```python
from build123d import *

# Parameters (mm, degrees)
SKETCH_1_R          = 17.5
EXTRUDE_1_DEPTH     = 15
SKETCH_2_R          = 1.5
CUT_EXTRUDE_1_DEPTH = 5
SKETCH_4_R          = 3
CUT_EXTRUDE_2_DEPTH = 20
SKETCH_5_R          = 1.5
CUT_EXTRUDE_3_DEPTH = 6
CHAMFER_1_SIZE      = 1.5
SKETCH_6_R          = 6.5
SKETCH_6_R_2        = 3.996615851
CUT_EXTRUDE_4_DEPTH = 3
SKETCH_7_R          = 3.996615851
SKETCH_7_R_2        = 3
EXTRUDE_2_DEPTH     = 1


with BuildPart() as part:
    # 草图1 → 凸台-拉伸1 (new body)
    with BuildSketch(Plane.XY):
        Circle(SKETCH_1_R)
    extrude(amount=EXTRUDE_1_DEPTH)

    # 草图2 → 切除-拉伸1 (cut)
    with BuildSketch(Plane(origin=(0, 0, 0), x_dir=(-1, 0, 0), z_dir=(0, 0, -1))):
        with Locations((0, -8)):
            Circle(SKETCH_2_R)
        with Locations((-8, 0)):
            Circle(SKETCH_2_R)
        with Locations((0, 8)):
            Circle(SKETCH_2_R)
        with Locations((8, 0)):
            Circle(SKETCH_2_R)
    extrude(amount=-CUT_EXTRUDE_1_DEPTH, mode=Mode.SUBTRACT)

    # 草图3 → 切除-旋转1 (revolve, cut)
    with BuildSketch(Plane(origin=(0, 0, 0), x_dir=(1, 0, 0), z_dir=(0, 1, 0))):
        Polygon((13.284433797, -10), (13.284433797, -9.953144571), (13.284433797, -9.453144571), (17.969347124, -9.453144571), (17.969347124, -10), align=None)
    revolve(axis=Axis((0, 0, 0), (0, 0, 1)), mode=Mode.SUBTRACT)

    # 草图4 → 切除-拉伸2 (cut)
    with BuildSketch(Plane(origin=(0, 0, 0), x_dir=(-1, 0, 0), z_dir=(0, 0, -1))):
        Circle(SKETCH_4_R)
    extrude(amount=-CUT_EXTRUDE_2_DEPTH, mode=Mode.SUBTRACT)

    # 草图5 → 切除-拉伸3 (cut)
    with BuildSketch(Plane.XY.offset(15)):
        with Locations((0, -9.5)):
            Circle(SKETCH_5_R)
        with Locations((-9.5, 0)):
            Circle(SKETCH_5_R)
        with Locations((0, 9.5)):
            Circle(SKETCH_5_R)
        with Locations((9.5, 0)):
            Circle(SKETCH_5_R)
    extrude(amount=-CUT_EXTRUDE_3_DEPTH, mode=Mode.SUBTRACT)

    # 倒角1
    chamfer_1_edges = [part.edges().sort_by_distance(p)[0] for p in [
        (-17.5, 0, 0),
        (-17.5, 0, 15),
    ]]
    chamfer(chamfer_1_edges, length=CHAMFER_1_SIZE)

    # 草图6 → 切除-拉伸4 (cut)
    with BuildSketch(Plane.XY.offset(15)):
        Circle(SKETCH_6_R)
        Circle(SKETCH_6_R_2, mode=Mode.SUBTRACT)
    extrude(amount=-CUT_EXTRUDE_4_DEPTH, mode=Mode.SUBTRACT)

    # 草图7 → 凸台-拉伸2 (add)
    with BuildSketch(Plane.XY.offset(15)):
        Circle(SKETCH_7_R)
        Circle(SKETCH_7_R_2, mode=Mode.SUBTRACT)
    extrude(amount=EXTRUDE_2_DEPTH)


solid = part.part
```
Check sheet for the modelled part. Datum: model origin and axes. Units: mm. A direction names the side the tool comes from. Round coordinates to 2 decimals unless told otherwise and drop trailing zeros. Order: outer loops, then holes, each group sorted by start corner. A loop starts at its lowest first (then second) coordinate and runs counter-clockwise, first axis right, second up. Notation, with made-up numbers: (3, 29.25) - (39, 29.25) arc R37 ccw to (39, 65.25) - close; hole circle Ø10 at (81.25, 53). An arc over 180 degrees is marked (long way). Answer as CSV lines item,"result". Start each with the question number.
1) Section check C-C (z = 6). Record the cut outline in (x, y).
2) Depth check by flat-ended pin: pin 1 (2.5 mm diameter, centred on x = 8, y = 0, fed in from -Z); pin 2 (4 mm diameter, centred on x = -8, y = 0, fed in from +Z); pin 3 (3 mm diameter, centred on x = -9.5, z = 10, fed in from +Y). Enter the tip coordinate at first touch or a pass-through.
3) Section check B-B (z = 4). Record the cut outline in (x, y), then the cut area to 3 significant figures.
4) Section check A-A (z = 14). Record the cut outline in (x, y).
5) Tool access check on faces 5 (the face through (12, 7, 10)), 6 (the face through (0, 8, 12)), 7 (the face through (0.325, 6.536, 2.465)), 8 (the face through (-0.2, -3.3, 0)), 9 (the face through (-13.887, -10.648, 5.421)). Record the directions out of +Z, -Z, +X, -X, +Y, -Y that give a thin tool (end or side, any length) a straight path to the whole face; none if there is none.
6) Scan lines: probe 1 along Y at (x, z) = (0, 12.6); probe 2 along Z at (x, y) = (-13, -8.5); probe 3 along Y at (x, z) = (1, 4). Record each from-to range of solid material in increasing order.
7) Draft check along X on faces 1 (the face through (8, 0, 5)), 2 (the face through (-13.887, -10.648, 11.726)), 3 (the face through (-12, 7, 9.453)), 4 (the face through (9, 0, 9)). Enter one of: +X half, -X half, draft (parallel to the pull), parting line (faces both ways), or undercut.
Determined:
1,outline,"circle Ø35 at (0, 0); hole circle Ø6 at (0, 0)"
2,pin 1,"z = 5"
2,pin 2,"z = 15"
2,pin 3,"y = 15.56"
3,outline,"circle Ø35 at (0, 0); hole circle Ø3 at (-8, 0); hole circle Ø6 at (0, 0); hole circle Ø3 at (0, -8); hole circle Ø3 at (0, 8); hole circle Ø3 at (8, 0)"
3,area,"906 mm^2"
4,outline,"circle Ø34 at (0, 0); circle Ø7.99 at (0, 0); hole circle Ø3 at (-9.5, 0); hole circle Ø13 at (0, 0); hole circle Ø6 at (0, 0); hole circle Ø3 at (0, -9.5); hole circle Ø3 at (0, 9.5); hole circle Ø3 at (9.5, 0)"
5,face 5,"none"
5,face 6,"+Z"
5,face 7,"-Z"
5,face 8,"-Z, +X, -X, +Y, -Y"
5,face 9,"+Z, -Z"
6,probe 1,"-17.5 to -11, -8 to -6.5, -4 to -3, 3 to 4, 6.5 to 8, 11 to 17.5"
6,probe 2,"0 to 9.45, 10 to 15"
6,probe 3,"-17.47 to -9.12, -6.88 to -2.83, 2.83 to 6.88, 9.12 to 17.47"
7,face 1,"undercut"
7,face 2,"parting line"
7,face 3,"draft"
7,face 4,"undercut"
